For this review, take the finished solid that the model builds, in its own axes (mm). Face numbers are marked on the shaded views. Coordinates: 2 decimals unless noted, no trailing zeros. Loops run counter-clockwise (first coordinate to the right, second up) from the corner with the lowest first, then second, coordinate; pieces in that order, holes last.
```python
from build123d import *

# Parameters (mm, degrees)
F5_W      = 10
F5_H      = 16
F6_DEPTH  = 5
F0_R      = 1.9
F2_R      = 1.9
F9_R      = 4.99999
F11_DEPTH = 0.2


# Not quite as in the source:
# - a fillet or chamfer is up to 0.001 mm smaller than in the source, because OpenCascade refuses the exact size


with BuildPart() as f6:
    # F5 (on offset) → F6 (new body)
    with BuildSketch(Plane.XY.offset(4.1)):
        with Locations((0, -95.8120375872)):
            Rectangle(F5_W, F5_H)
    extrude(amount=-F6_DEPTH)

    # F0 (on Front) → F7 (revolve, cut)
    with BuildSketch(Plane.XZ):
        with Locations((-92.5, 0)):
            Circle(F0_R)
    revolve(axis=Axis((0, 0, 0), (0, 0, 1)), mode=Mode.SUBTRACT)

    # F2 (on Front) → F8 (revolve, cut)
    with BuildSketch(Plane.XZ):
        with Locations((-100, 0)):
            Circle(F2_R)
    revolve(axis=Axis((0, 0, 0), (0, 0, 1)), mode=Mode.SUBTRACT)

    # F9 (radius 5 in the source; OpenCascade refuses exactly that, so slightly less here)
    f9_edges = [f6.edges().sort_by_distance(p)[0] for p in [
        (0, -103.812038, 4.1),
        (0, -87.812038, 4.1),
    ]]
    fillet(f9_edges, radius=F9_R)

    # F10 (on face) → F11 (join)
    with BuildSketch(Plane.YZ.offset(5)):
        with BuildLine():
            Line((-92.8120375872, 4.1), (-98.8120375872, 4.1))
            ThreePointArc((-98.8120375872, 4.1), (-102.3475714931, 2.6355339059), (-103.8120375872, -0.9))
            Line((-103.8120375872, -0.9), (-87.8120375872, -0.9))
            ThreePointArc((-87.8120375872, -0.9), (-89.2765036812, 2.6355339059), (-92.8120375872, 4.1))
        make_face()
    extrude(amount=-F11_DEPTH)


solid = f6.part
```
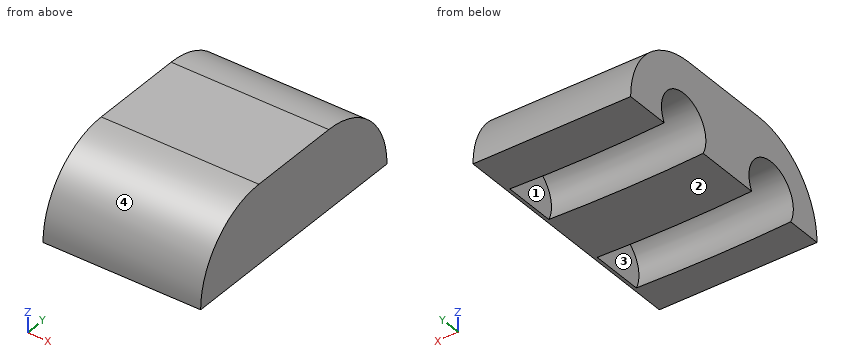
Q1. Wall thickness on probe 1 along Y at (x, z) = (0.5, 0.35); probe 2 along Y at (x, z) = (4.25, 0.9); probe 3 along X at (y, z) = (-93, 0.65): over which ranges is each line inside the solid? List them lowest first.
Q2. The part is to be moulded in two halves that separate along Y. For the marked faces 1, 2, 3 and 4, say which applies: +Y half, -Y half, draft (parallel to the pull), parting line (faces both ways), or undercut.
Q3. Consider section A-A (z = -0.1). State the section outline as (x, y) points, then the cut area to 3 significant figures.
Q4. For pin 1 Ø2 at (y, z) = (-99.5, 0) entering from -X; pin 2 Ø1.5 at (x, z) = (-2.5, 1) entering from +Y, all flat-tipped, find the tip position at first contact; note any pin that passes through.
Q5. Consider section C-C (z = 1.1). State the section outline as (x, y) points.
Q6. Consider section D-D (z = 3.3). State the section outline as (x, y) points.
Q7. Consider section B-B (y = -89). State the section outline as (x, z) points.
Model answer:
1. probe 1: y = -103.65 to -101.87, -98.13 to -94.37, -90.63 to -87.97
1. probe 2: y = -103.48 to -101.58, -98.23 to -94.08, -90.73 to -88.15
1. probe 3: x = 4.8 to 5
2. face 1: undercut
2. face 2: draft
2. face 3: undercut
2. face 4: -Y half
3. outline: (-5, -103.75) - (5, -103.75) - (5, -87.88) - (-5, -87.88) - (-5, -90.46) arc R90.6 ccw to (4.8, -90.48) - (4.8, -94.28) arc R94.4 cw to (-5, -94.26) - (-5, -97.98) arc R98.1 ccw to (4.8, -97.99) - (4.8, -101.78) arc R101.9 cw to (-5, -101.77) - close
3. area: 84.3 mm2
4. pin 1: stops at x = 4.8
4. pin 2: stops at y = -87.95
5. outline: (-5, -103.39) - (5, -103.39) - (5, -88.23) - (-5, -88.23) - (-5, -90.81) arc R90.95 ccw to (4.8, -90.82) - (4.8, -93.93) arc R94.05 cw to (-5, -93.92) - (-5, -98.32) arc R98.45 ccw to (4.8, -98.33) - (4.8, -101.44) arc R101.55 cw to (-5, -101.43) - close
6. outline: (-5, -101.52) - (5, -101.52) - (5, -90.1) - (-5, -90.1) - close
7. outline: (-5, -0.9) - (5, -0.9) - (5, 2.34) - (-5, 2.34) - close
